from build123d import *

# Parameters (mm, degrees)
F0_W     = 100
F0_H     = 100
F1_DEPTH = 10
F2_R     = 5
F3_DEPTH = 15
F4_DEPTH = 17.5


with BuildPart() as f1:
    # F0 (on Front) → F1 (new body)
    with BuildSketch(Plane.XZ):
        Rectangle(F0_W, F0_H)
    extrude(amount=-F1_DEPTH)

    # F2 (on face) → F3 (join)
    with BuildSketch(Plane.XZ):
        with Locations((-20, 0)):
            Circle(F2_R)
        with BuildLine():
            ThreePointArc((13.07182, 2.150912), (8.872353, 3.576439), (6.25, 0))
            Line((6.25, 0), (10, 0))
            Line((10, 0), (13.07182, 2.150912))
        make_face()
        with BuildLine():
            Line((10, 0), (6.25, 0))
            ThreePointArc((6.25, 0), (10, -3.75), (13.75, 0))
            ThreePointArc((13.75, 0), (13.576439, 1.127647), (13.07182, 2.150912))
            Line((13.07182, 2.150912), (10, 0))
        make_face()
    extrude(amount=F3_DEPTH)

    # F2 (on face) → F4 (join)
    with BuildSketch(Plane.XZ):
        with BuildLine():
            ThreePointArc((24.787281, 8.603647), (21.535516, 10.987939), (20.239401, 7.169705))
            ThreePointArc((20.239401, 7.169705), (23.039045, 6.219354), (24.787281, 8.603647))
        make_face()
    extrude(amount=F4_DEPTH)


solid = f1.part
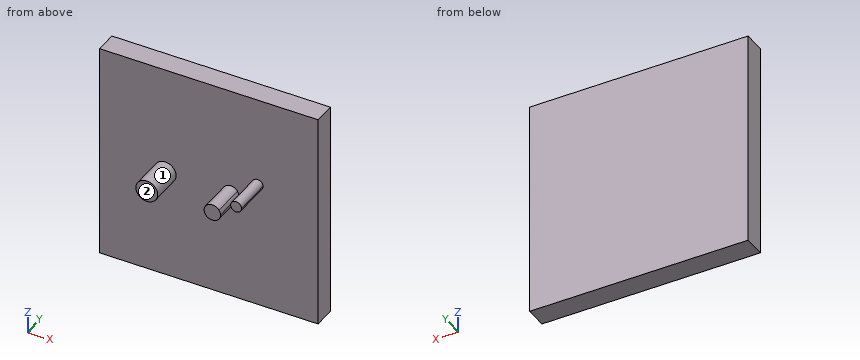
Can you work these out from the model? Positions are in its coordinate system, mm. Face numbers are marked on the shaded views. Coordinates: 2 decimals unless noted, no trailing zeros. Loops run counter-clockwise (first coordinate to the right, second up) from the corner with the lowest first, then second, coordinate; pieces in that order, holes last. Notation, with made-up numbers: (-18, 35) - (11, 35) arc R20 cw to (11, 62) - close; hole circle Ø3 at (23, 57). An arc over 180 degrees is marked (long way). Answer as a JSON object with one key per item and string values. Group by question number.
Item 1: If we section it at D-D (x = -20): List the corners of the cut face in (y, z) for me, plus the area to 3 significant figures.
Item 2: If we section it at A-A (y = -13): List the corners of the cut face in (x, z) for me, plus the area to 3 significant figures.
Item 3: If we section it at C-C (z = -29): List the corners of the cut face in (x, y) for me.
Item 4: If I drill on L1, parallel to Y at x = -19, z = 23; L2, parallel to Z at x = 22, y = -10.75; L3, parallel to X at y = -11.5, z = -0.5, over which ranges is the centre line in solid material (lowest first)? Write a range as from..to.
Item 5: For pin 1 (1 mm diameter, centred on x = -16, z = -11.5, fed in from -Y); pin 2 (11 mm diameter, centred on x = -18, z = 1.5, fed in from -Y); pin 3 (5 mm diameter, centred on x = -26.5, y = -6, fed in from +Z); pin 4 (12 mm diameter, centred on x = 39.5, y = -11.5, fed in from +Z), each with a flat end and sliding along its axis, tell me the tip position at first contact or that it passes through.
Item 6: If we mould it in two halves opening along X, with no side actions, what happens to the marked faces 1 and 2? For each: released by +X, released by -X, zero draft, split by the parting line, or undercut.
Item 7: If we section it at B-B (x = 10): List the corners of the cut face in (y, z) for me.
Returned:
{
 "1": {"outline": "(-15, -5) - (0, -5) - (0, -50) - (10, -50) - (10, 50) - (0, 50) - (0, 5) - (-15, 5) - close", "area": "1,150 mm²"},
 "2": {"outline": "circle Ø10 at (-20, 0); (13.07, 2.15) arc R3.75 ccw (long way) to (13.75, 0) arc R3.75 ccw to start; circle Ø5 at (22.29, 8.6)", "area": "142 mm²"},
 "3": {"outline": "(-50, 0) - (50, 0) - (50, 10) - (-50, 10) - close"},
 "4": {"L1": "y = 0..10", "L2": "z = 6.12..11.09", "L3": "x = -24.97..-15.03, 6.28..13.72"},
 "5": {"pin 1": "stops at y = 0", "pin 2": "stops at y = -15", "pin 3": "stops at z = 3", "pin 4": "passes through"},
 "6": {"face 1": "undercut", "face 2": "zero draft"},
 "7": {"outline": "(-15, -3.75) - (0, -3.75) - (0, -50) - (10, -50) - (10, 50) - (0, 50) - (0, 3.75) - (-15, 3.75) - close"}
}
